from build123d import *

# Parameters (mm, degrees)
F0_W     = 146
F0_H     = 4
F1_DEPTH = 175
F3_DEPTH = 4
F5_DEPTH = 4


with BuildPart() as f1:
    # F0 (on Right) → F1 (new body, symmetric)
    with BuildSketch(Plane.YZ):
        with Locations((-73, 2)):
            Rectangle(F0_W, F0_H)
    extrude(amount=F1_DEPTH, both=True)

    # F2 (on face) → F3 (cut, through all)
    with BuildSketch(Plane.XY.offset(4)):
        Polygon((-175, 0), (-175, -146), (12.940962, 0), align=None)
        Polygon((55.940962, 0), (175, -146), (175, 0), align=None)
    extrude(amount=-F3_DEPTH, mode=Mode.SUBTRACT)

    # F4 (on face) → F5 (cut, through all)
    with BuildSketch(Plane.XY.offset(4)):
        Polygon((55.940962, 0), (12.940962, 0), (76.425021, -25.119241), align=None)
    extrude(amount=-F5_DEPTH, mode=Mode.SUBTRACT)


solid = f1.part
For this review, take the finished solid that the model builds, in its own axes (mm). Round coordinates to 2 decimals unless told otherwise and drop trailing zeros. Loops run counter-clockwise (first coordinate to the right, second up) from the corner with the lowest first, then second, coordinate; pieces in that order, holes last. Notation, with made-up numbers: (38.25, 12.5) - (73.25, 12.5) arc R20 cw to (73.25, 41.5) - close; hole circle Ø11 at (30.5, 38.5). An arc over 180 degrees is marked (long way). Put each result on its own line as item: value. Start each with the question number.
1. For probe 1 along X at (y, z) = (-113, 3.35); probe 2 along Y at (x, z) = (29.5, 3.3); probe 3 along Y at (x, z) = (-80, 2.1), list the stretches that pass through material, from the lowest coordinate up. Write a range as [from, to].
2. Consider section B-B on x = -36.5. State the section outline as (y, z) points.
3. Consider section A-A on z = 3.05. State the section outline as (x, y) points.
4. Insertion check: P1, Ø1, axis at x = -33, y = -79, coming from the -Z side. The pin has a flat end and moves straight along its axis. Give the tip position at first contact, or say it passes through.
Result sheet:
1. probe 1: [-132.52, 148.09]
1. probe 2: [-146, -6.55]
1. probe 3: [-146, -72.2]
2. outline: (-146, 0) - (-38.41, 0) - (-38.41, 4) - (-146, 4) - close
3. outline: (-175, -146) - (175, -146) - (76.43, -25.12) - (12.94, 0) - close
4. P1: z = 0
